Design review of the part shown in the three views and the two pictorial views. Dimensions are in mm from the part's minimum x, y and z. A direction names the side the tool comes from. Coordinates: 2 decimals unless noted, no trailing zeros. Loops run counter-clockwise (first coordinate to the right, second up) from the corner with the lowest first, then second, coordinate; pieces in that order, holes last. Notation, with made-up numbers: (-27, 10.25) -> (-10, 10.25) arc R14 cw to (-10, 22.25) -> close; hole circle Ø2 at (77.25, 23.25). An arc over 180 degrees is marked (long way). One line per item, written item: value.
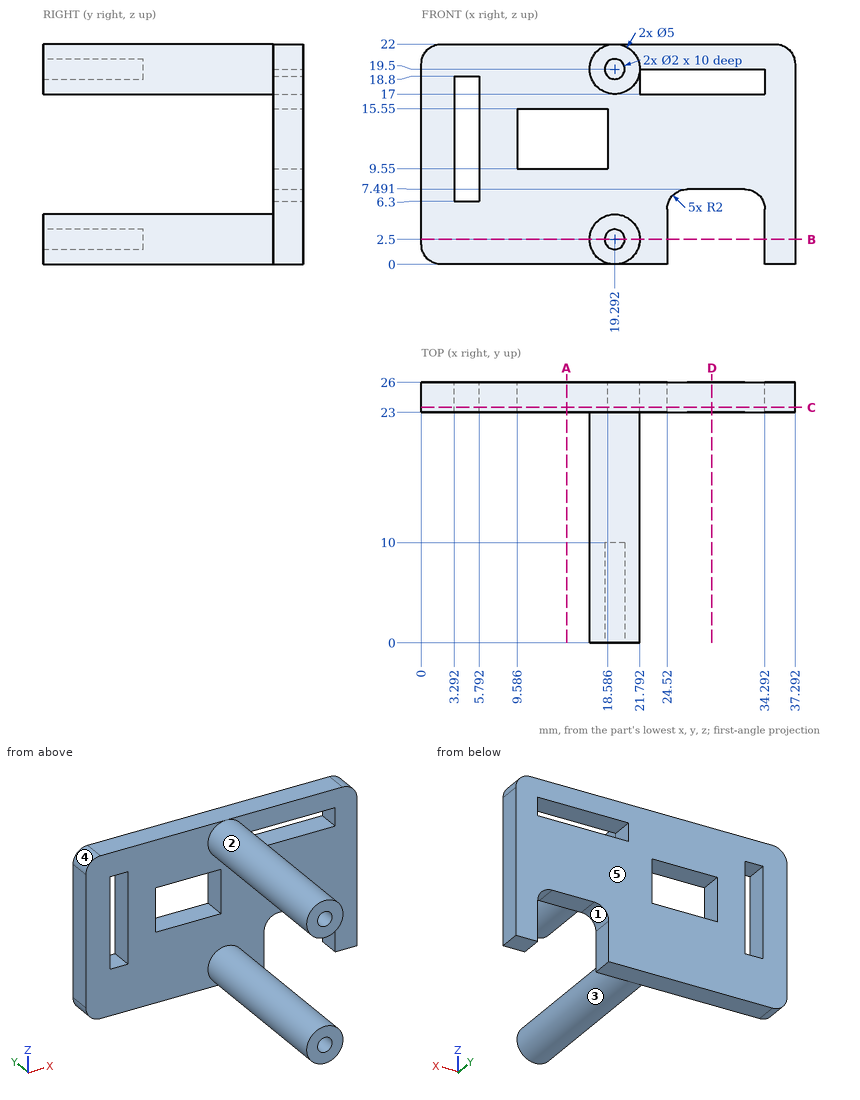
1. The part is to be moulded in two halves that separate along Z. For the marked faces 3, 4 and 5, say which applies: pulls with the +Z half, pulls with the -Z half, needs draft (parallel to the pull), parting line crosses it, or undercut.
Return value:
face 3: undercut
face 4: pulls with the +Z half
face 5: needs draft
2. Take a section at C-C, the plane y = 23.5. Give the number of separate pieces and of enclosed holes in the cut face, and give its area (3 significant figures).
Return value:
separate pieces: 1
enclosed holes: 3
area: 630 mm2
3. To check wall thickness, follow probe 1 along X at (y, z) = (4, 2.5); probe 2 along Z at (x, y) = (19.5, 8); probe 3 along Z at (x, y) = (4, 23.5). State the ranges of each line that lie inside material, in increasing order. Write a range as from..to.
Return value:
probe 1: x = 16.79..18.29, 20.29..21.79
probe 2: z = 0.01..1.52, 3.48..4.99, 17.01..18.52, 20.48..21.99
probe 3: z = 0..6.3, 18.8..22
4. Take a section at D-D, the plane x = 29. Give the boundary of the cut face in (y, z).
Return value:
outline: (23, 7.49) -> (26, 7.49) -> (26, 17) -> (23, 17) -> close; (23, 19.5) -> (26, 19.5) -> (26, 22) -> (23, 22) -> close
5. Take a section at A-A, the plane x = 14.5. Give the boundary of the cut face in (y, z), and give its area (3 significant figures).
Return value:
outline: (23, 0) -> (26, 0) -> (26, 9.55) -> (23, 9.55) -> close; (23, 15.55) -> (26, 15.55) -> (26, 22) -> (23, 22) -> close
area: 48.0 mm2
6. Insertion check: pin 1 Ø0.6 at (x, z) = (19.5, 20) entering from -Y; pin 2 Ø2 at (y, z) = (16, 4.5) entering from -X; pin 3 Ø1.5 at (x, y) = (16.5, 3.5) entering from +Z (1 decimal); pin 4 Ø1 at (x, z) = (15.5, 15) entering from -Y. Each pin has a flat end and moves straight along its axis. Give the tip position at first contact, or say it passes through.
Return value:
pin 1: stops at y = 10
pin 2: stops at x = 17
pin 3: stops at z = 20.9
pin 4: passes through
7. For the marked faces 1 and 2, list the 3-axis set-ups (+Z, -Z, +X, -X, +Y, -Y) from which the entire face can be reached by the end or side of a thin tool; tool diameter is ignored.
Return value:
face 1: -Z, +Y, -Y
face 2: -Y
8. Take a section at B-B, the plane z = 2.5. Give the boundary of the cut face in (x, y).
Return value:
outline: (0, 23) -> (16.79, 23) -> (16.79, 0) -> (18.29, 0) -> (18.29, 10) -> (20.29, 10) -> (20.29, 0) -> (21.79, 0) -> (21.79, 23) -> (24.52, 23) -> (24.52, 26) -> (0, 26) -> close; (34.29, 23) -> (37.29, 23) -> (37.29, 26) -> (34.29, 26) -> close
